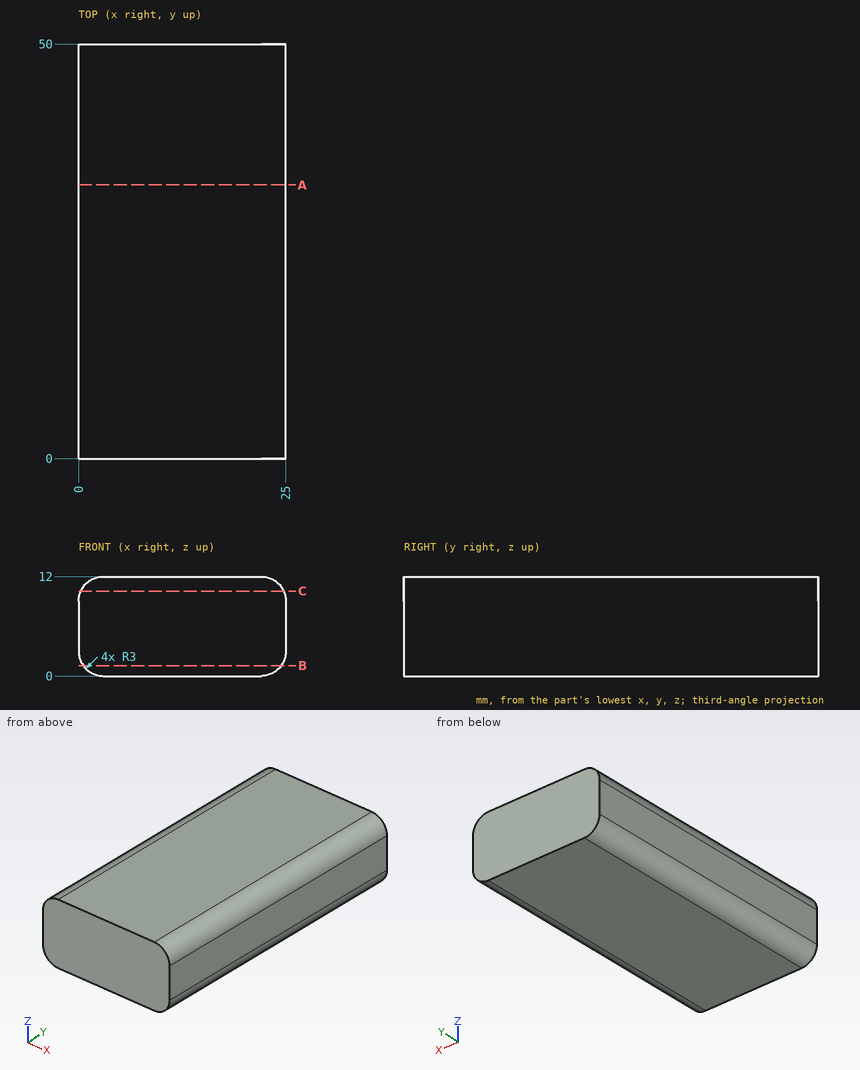
Source: three-view drawing plus pictorial views. Frame: mm from the lowest corner of the part. Coordinates: 2 decimals unless noted, no trailing zeros. Write each loop counter-clockwise with the first axis right and the second up, starting at its lowest first coordinate (ties: lowest second). Pieces come first, ordered by that corner, then holes. Notation, with made-up numbers: (-17.5, 18.25) - (12.5, 18.25) arc R9 cw to (12.5, 28.25) - close; hole circle Ø11 at (68, 67). An arc over 180 degrees is marked (long way). Return JSON: item names as keys, results as strings.
Item 1: Line query: L1, parallel to Z at x = 2.75, y = 13; L2, parallel to Z at x = 2, y = 32.5; L3, parallel to X at y = 16.5, z = 10.5. Output: solid intervals per line, ascending.
Completed:
{"L1": "z = 0.01 to 11.99", "L2": "z = 0.17 to 11.83", "L3": "x = 0.4 to 24.6"}
Item 2: Section query C-C (z = 10.25). Output: boundary loops of the cut face in (x, y), and give its area (3 significant figures).
Completed:
{"outline": "(0.27, 0) - (24.73, 0) - (24.73, 50) - (0.27, 50) - close", "area": "1,220 mm2"}
Item 3: Section query B-B (z = 1.25). Output: boundary loops of the cut face in (x, y).
Completed:
{"outline": "(0.56, 0) - (24.44, 0) - (24.44, 50) - (0.56, 50) - close"}
Item 4: Section query A-A (y = 33). Output: boundary loops of the cut face in (x, z).
Completed:
{"outline": "(0, 3) arc R3 ccw to (3, 0) - (22, 0) arc R3 ccw to (25, 3) - (25, 9) arc R3 ccw to (22, 12) - (3, 12) arc R3 ccw to (0, 9) - close"}
